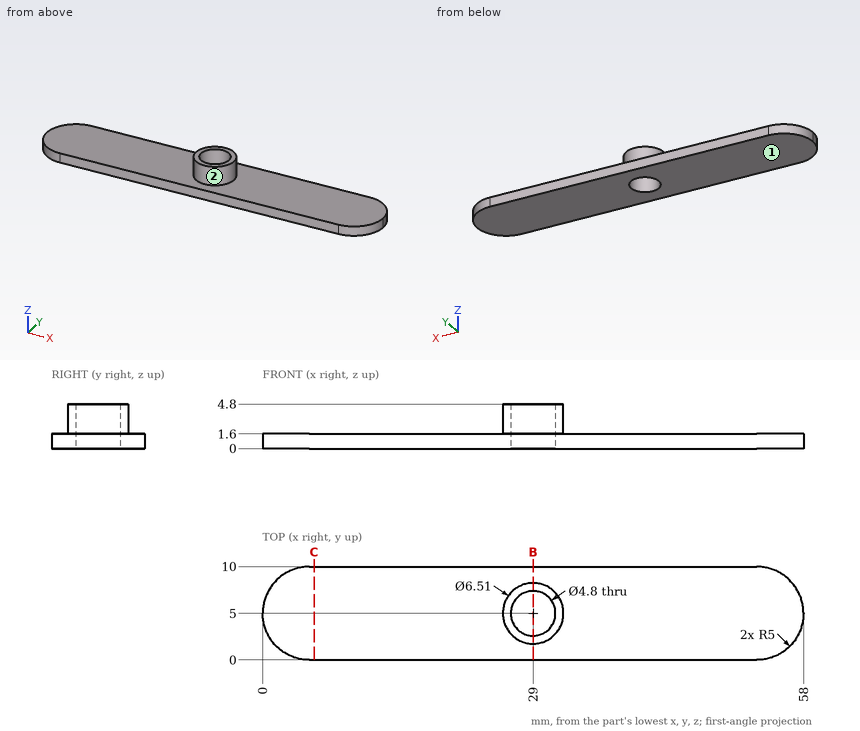
Print and shaded views of the part. All mm, measured from the part's lowest x, y and z. A direction names the side the tool comes from. Coordinates: 2 decimals unless noted, no trailing zeros. Order: outer loops, then holes, each group sorted by start corner. A loop starts at its lowest first (then second) coordinate and runs counter-clockwise, first axis right, second up.
Item 1: Drill centre lines: L1, parallel to Y at x = 29, z = 2.45 (3 decimals); L2, parallel to Z at x = 19.5, y = 7; L3, parallel to X at y = 7, z = 3.75. Where is each one in solid material? Low to high.
Filled in:
L1: y = 1.745 to 2.6, 7.4 to 8.255
L2: z = 0 to 1.6
L3: x = 26.43 to 27.67, 30.33 to 31.57
Item 2: Saw through at B-B on x = 29. List the corners of the cut face in (y, z) (3 decimals), then the cut area to 3 significant figures.
Filled in:
outline: (0, 0) - (2.6, 0) - (2.6, 4.8) - (1.745, 4.8) - (1.745, 1.6) - (0, 1.6) - close; (7.4, 0) - (10, 0) - (10, 1.6) - (8.255, 1.6) - (8.255, 4.8) - (7.4, 4.8) - close
area: 13.8 mm2
Item 3: Tool access for the marked faces 1 and 2: list every direction of +Z, -Z, +X, -X, +Y, -Y with a clear straight run to the whole face (end or side of a thin tool).
Filled in:
face 1: -Z, +X, -X, +Y, -Y
face 2: +Z
Item 4: Drop a flat-ended pin along its axis: pin 1 Ø3 at (x, y) = (29, 5) entering from -Z. Give the stop position or say it passes through.
Filled in:
pin 1: passes through
Item 5: Saw through at C-C on x = 5.5. List the corners of the cut face in (y, z).
Filled in:
outline: (0, 0) - (10, 0) - (10, 1.6) - (0, 1.6) - close
